```python
from build123d import *

# Parameters (mm, degrees)
SKETCH1_R           = 75
SKETCH1_R_2         = 27
SKETCH1_R_3         = 5
SKETCH1_R_4         = 4
BOSS_EXTRUDE1_DEPTH = 10


with BuildPart() as part:
    # Sketch1 → Boss-Extrude1 (new body)
    with BuildSketch(Plane.XY):
        Circle(SKETCH1_R)
        with Locations((-29.69848481, 29.69848481)):
            Circle(SKETCH1_R_2, mode=Mode.SUBTRACT)
        with Locations((29.69848481, 29.69848481)):
            Circle(SKETCH1_R_2, mode=Mode.SUBTRACT)
        with Locations((29.69848481, -29.69848481)):
            Circle(SKETCH1_R_2, mode=Mode.SUBTRACT)
        with Locations((-29.69848481, -29.69848481)):
            Circle(SKETCH1_R_2, mode=Mode.SUBTRACT)
        Circle(SKETCH1_R_3, mode=Mode.SUBTRACT)
        with Locations((0, 65)):
            Circle(SKETCH1_R_4, mode=Mode.SUBTRACT)
        with Locations((65, 0)):
            Circle(SKETCH1_R_4, mode=Mode.SUBTRACT)
        with Locations((0, -65)):
            Circle(SKETCH1_R_4, mode=Mode.SUBTRACT)
        with Locations((-65, 0)):
            Circle(SKETCH1_R_4, mode=Mode.SUBTRACT)
    extrude(amount=BOSS_EXTRUDE1_DEPTH)


solid = part.part
```
Input: part model. Units: mm. Frame: model coordinates. Give positions to 0.01 mm unless a question says otherwise; leave off trailing zeros. Write each loop counter-clockwise with the first axis right and the second up, starting at its lowest first coordinate (ties: lowest second). Pieces come first, ordered by that corner, then holes. Notation, with made-up numbers: (21.25, 48) - (78.25, 48) arc R36 cw to (78.25, 86) - close; hole circle Ø4 at (-33.75, -24). An arc over 180 degrees is marked (long way). Write item = value, one per line. Start each with the question number.
1) Cut plane B-B (x = -0.5). Return loops of the section in (y, z), and give its area (3 significant figures).
2) Cut plane C-C (y = 0). Return loops of the section in (x, z).
3) Material intervals for L1, parallel to Y at x = 0, z = 6.25; L2, parallel to X at y = 44.5, z = 6; L3, parallel to Y at x = 15.5, z = 5.5, sorted ascending. Write a range as [from, to].
4) Cut plane D-D (x = 66.5). Return loops of the section in (y, z).
5) Draft query along X for faces 1 (the face through (-0.867, 61.095, 4.93)), 2 (the face through (-0.4, -5.2, 0)), 3 (the face through (-9.764, 74.362, 4.93)). Return one class per face: pulls with the +X half, pulls with the -X half, needs draft (parallel to the pull), parting line crosses it, or undercut.
6) Cut plane A-A (y = 45). Return loops of the section in (x, z), and give its area (3 significant figures).
7) Pin query (flat end, axial travel): pin 1 (4 mm diameter, centred on y = -27, z = 7.5, fed in from -X); pin 2 (1.5 mm diameter, centred on y = 20.5, z = 6, fed in from -X); pin 3 (1.5 mm diameter, centred on y = 35.5, z = 9, fed in from -X); pin 4 (7 mm diameter, centred on x = 65, y = 0, fed in from -Z). Return the tip coordinate at first contact, or that it passes through.
Answers follow:
q1.outline = (-75, 0) - (-68.97, 0) - (-68.97, 10) - (-75, 10) - close; (-61.03, 0) - (-4.97, 0) - (-4.97, 10) - (-61.03, 10) - close; (4.97, 0) - (61.03, 0) - (61.03, 10) - (4.97, 10) - close; (68.97, 0) - (75, 0) - (75, 10) - (68.97, 10) - close
q1.area = 1,240 mm^2
q2.outline = (-75, 0) - (-69, 0) - (-69, 10) - (-75, 10) - close; (-61, 0) - (-5, 0) - (-5, 10) - (-61, 10) - close; (5, 0) - (61, 0) - (61, 10) - (5, 10) - close; (69, 0) - (75, 0) - (75, 10) - (69, 10) - close
q3.L1 = [-75, -69], [-61, -5], [5, 61], [69, 75]
q3.L2 = [-60.37, -52.28], [-7.12, 7.12], [52.28, 60.37]
q3.L3 = [-73.38, -52.66], [-6.73, 6.73], [52.66, 73.38]
q4.outline = (-34.68, 0) - (-3.71, 0) - (-3.71, 10) - (-34.68, 10) - close; (3.71, 0) - (34.68, 0) - (34.68, 10) - (3.71, 10) - close
q5.face_1 = undercut
q5.face_2 = needs draft
q5.face_3 = parting line crosses it
q6.outline = (-60, 0) - (-51.94, 0) - (-51.94, 10) - (-60, 10) - close; (-7.45, 0) - (7.45, 0) - (7.45, 10) - (-7.45, 10) - close; (51.94, 0) - (60, 0) - (60, 10) - (51.94, 10) - close
q6.area = 310 mm^2
q7.pin_1 = -70.71
q7.pin_2 = -72.35
q7.pin_3 = -66.46
q7.pin_4 = through
